```python
from build123d import *

# Parameters (mm, degrees)
BOSS_EXTRUDE1_DEPTH = 5


with BuildPart() as part:
    # Sketch1 → Boss-Extrude1 (new body)
    with BuildSketch(Plane.XY):
        Polygon((-7.5, 40), (-7.5, 45), (-2.5, 45), (-2.5, 40), (2.5, 40), (2.5, 45), (7.5, 45), (7.5, 40), (10, 40), (10, -40), (7.5, -40), (7.5, -50), (2.5, -50), (2.5, -45), (2.5, -40), (-2.5, -40), (-2.5, -50), (-7.5, -50), (-7.5, -45), (-7.5, -40), (-10, -40), (-10, 40), align=None)
        with BuildLine():
            Line((3, -11.2), (3, -5))
            ThreePointArc((3, -5), (4, -4), (5, -5))
            Line((5, -5), (5, -11.2))
            ThreePointArc((5, -11.2), (4, -12.2), (3, -11.2))
        make_face(mode=Mode.SUBTRACT)
        with BuildLine():
            Line((3, 11.2), (3, 5))
            ThreePointArc((3, 5), (4, 4), (5, 5))
            Line((5, 5), (5, 11.2))
            ThreePointArc((5, 11.2), (4, 12.2), (3, 11.2))
        make_face(mode=Mode.SUBTRACT)
        with BuildLine():
            Line((-3, 11.2), (-3, 5))
            ThreePointArc((-3, 5), (-4, 4), (-5, 5))
            Line((-5, 5), (-5, 11.2))
            ThreePointArc((-5, 11.2), (-4, 12.2), (-3, 11.2))
        make_face(mode=Mode.SUBTRACT)
        with BuildLine():
            Line((-3, -11.2), (-3, -5))
            ThreePointArc((-3, -5), (-4, -4), (-5, -5))
            Line((-5, -5), (-5, -11.2))
            ThreePointArc((-5, -11.2), (-4, -12.2), (-3, -11.2))
        make_face(mode=Mode.SUBTRACT)
    extrude(amount=BOSS_EXTRUDE1_DEPTH)


solid = part.part
```
For this review, take the finished solid that the model builds, in its own axes (mm). A direction names the side the tool comes from. Give positions to 0.01 mm unless a question says otherwise; leave off trailing zeros. Write each loop counter-clockwise with the first axis right and the second up, starting at its lowest first coordinate (ties: lowest second). Pieces come first, ordered by that corner, then holes. Notation, with made-up numbers: M 85.5,45 L 114.5,45 A20 ccw 114.5,65 Z; hole C -27.5,12.25 d7. An arc over 180 degrees is marked long. One line per item, written item: value.
1) For faces 5 (the cylindrical face through (4, -4, 2)), 6 (the flat face through (0, 40, 2)), 7 (the flat face through (9, -40, 2)), list the 3-axis set-ups (+Z, -Z, +X, -X, +Y, -Y) from which the entire face can be reached by the end or side of a thin tool; tool diameter is ignored.
Results are:
face 5: +Z, -Z
face 6: +Z, -Z, +Y
face 7: +Z, -Z, +X, -Y
2) Take a section at A-A, the plane y = 6. Write out the cut boundary in (x, z), then the cut area to 3 significant figures.
Results are:
outline: M -10,0 L -5,0 L -5,5 L -10,5 Z; M -3,0 L 3,0 L 3,5 L -3,5 Z; M 5,0 L 10,0 L 10,5 L 5,5 Z
area: 80.0 mm²
3) For P1, Ø2.5, axis at y = 42, z = 1.5, coming from the +X side; P2, Ø1.5, axis at x = 0, z = 2.5, coming from the +Y side; P3, Ø2.5, axis at y = 42.5, z = 1.5, coming from the -X side, all flat-tipped, find the tip position at first contact; note any pin that passes through.
Results are:
P1: stops at x = 7.5
P2: stops at y = 40
P3: stops at x = -7.5
4) Take a section at D-D, the plane z = 0.75. Count the separate pieces of the cut face and the enclosed holes in it, then the cut area to 3 significant figures.
Results are:
separate pieces: 1
enclosed holes: 4
area: 1,690 mm²
5) Take a section at C-C, the plane x = 8.75. Write out the cut boundary in (y, z), then the cut area to 3 significant figures.
Results are:
outline: M -40,0 L 40,0 L 40,5 L -40,5 Z
area: 400 mm²
6) The part is to be moulded in two halves that separate along X. For faces 1 (the cylindrical face through (-4, 4, 2)), 2 (the flat face through (-7.5, -45, 2)), 3 (the flat face through (-5, -50, 2)), 4 (the flat face through (0, -40, 2)), say which applies: +X half, -X half, draft (parallel to the pull), parting line (faces both ways), or undercut.
Results are:
face 1: undercut
face 2: -X half
face 3: draft
face 4: undercut
7) For line 1 (X direction, y = 10.5, z = 3.2); line 2 (X direction, y = -44, z = 3.05); line 3 (Y direction, x = 3.75, z = 0.2), list the stretches that pass through material, from the lowest coordinate up. Write a range as from..to.
Results are:
line 1: x = -10..-5, -3..3, 5..10
line 2: x = -7.5..-2.5, 2.5..7.5
line 3: y = -50..-12.17, -4.03..4.03, 12.17..45
8) Take a section at B-B, the plane x = -4. Write out the cut boundary in (y, z).
Results are:
outline: M -50,0 L -12.2,0 L -12.2,5 L -50,5 Z; M -4,0 L 4,0 L 4,5 L -4,5 Z; M 12.2,0 L 45,0 L 45,5 L 12.2,5 Z
